from build123d import *

# Parameters (mm, degrees)
FILLET1_R      = 0.79375
CHAMFER1_SIZE  = 0.79375
CHAMFER1_SIZE2 = 1.374815329


with BuildPart() as part:
    # Sketch1 → Revolve1 (revolve)
    with BuildSketch(Plane.XY):
        Polygon((0, 0), (-9.4234, 0), (-9.4234, 3.175), (-8.4836, 4.572), (-8.4836, 6.35), (-9.4234, 6.35), (-9.4234, 12.7), (0, 12.7), align=None)
    revolve(axis=Axis((0, 0, 0), (0, 1, 0)))

    # Fillet1
    fillet1_edges = [part.edges().sort_by_distance(p)[0] for p in [
        (9.4234, 0, 0),
    ]]
    fillet(fillet1_edges, radius=FILLET1_R)

    # Chamfer1
    chamfer1_edges = [part.edges().sort_by_distance(p)[0] for p in [
        (9.4234, 12.7, 0),
    ]]
    chamfer1_side = [part.faces().sort_by_distance(p)[0] for p in [
        (0, 12.7, 0),
    ]]
    chamfer(chamfer1_edges, length=CHAMFER1_SIZE, length2=CHAMFER1_SIZE2, reference=chamfer1_side[0])


solid = part.part
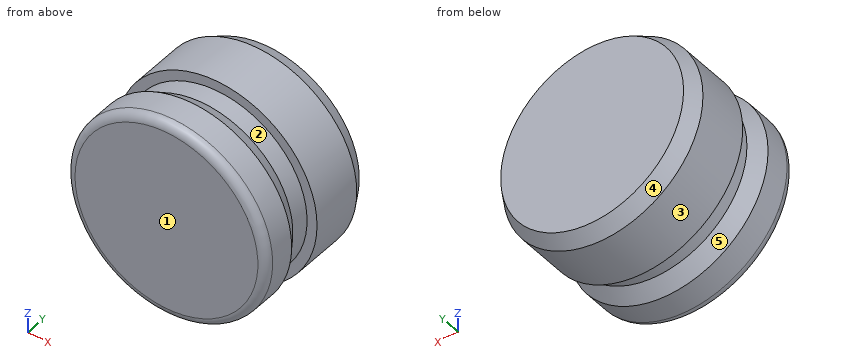
Verification items for the finished model (mm, model axes). Face numbers are marked on the shaded views. A direction names the side the tool comes from. Coordinates: 2 decimals unless noted, no trailing zeros. Write each loop counter-clockwise with the first axis right and the second up, starting at its lowest first coordinate (ties: lowest second). Pieces come first, ordered by that corner, then holes. Notation, with made-up numbers: M 75,79 L 94,79 A14 cw 94,89 Z; hole C 88.5,-23.75 d7. An arc over 180 degrees is marked long. Use a Markdown table: item, result.
Q1. Sectioned sample at D-D, the plane y = 6.75. Record the boundary of the cut face in (x, z).
Reply:
| item | result |
|---|---|
| outline | C 0,0 d18.85 |
Q2. Thickness scan on line 1 (Y direction, x = 5.25, z = -6.75); line 2 (Z direction, x = 0.25, y = 5.5); line 3 (Z direction, x = 0, y = 8.5). Record the ranges inside material, lowest first.
Reply:
| item | result |
|---|---|
| line 1 | y = 0 to 4.47, 6.35 to 12.7 |
| line 2 | z = -8.48 to 8.48 |
| line 3 | z = -9.42 to 9.42 |
Q3. Set-up check for the marked faces 4 and 5: record each of +Z, -Z, +X, -X, +Y, -Y from which the full face is reachable in a straight line by a thin tool's end or side.
Reply:
| item | result |
|---|---|
| face 4 | +Y |
| face 5 | none |
Q4. Sectioned sample at C-C, the plane y = 5.25. Record the boundary of the cut face in (x, z), plus the area to 3 significant figures.
Reply:
| item | result |
|---|---|
| outline | C 0,0 d16.97 |
| area | 226 mm² |
Q5. Draft check along Y on the marked faces 1, 2 and 3. Enter one of: +Y half, -Y half, draft (parallel to the pull), parting line (faces both ways), or undercut.
Reply:
| item | result |
|---|---|
| face 1 | -Y half |
| face 2 | undercut |
| face 3 | draft |
Q6. Go/stop test with flat-tipped pins: P1, Ø4, axis at x = 3.5, y = 7.5, coming from the +Z side; P2, Ø5.5, axis at x = -1.5, z = 3, coming from the -Y side; P3, Ø2, axis at y = 8, z = -6.5, coming from the -X side; P4, Ø2, axis at y = 2.5, z = -6.5, coming from the +X side. Record where each tip stops, or that it passes through.
Reply:
| item | result |
|---|---|
| P1 | stops at z = 9.3 |
| P2 | stops at y = 0 |
| P3 | stops at x = -7.65 |
| P4 | stops at x = 7.65 |
